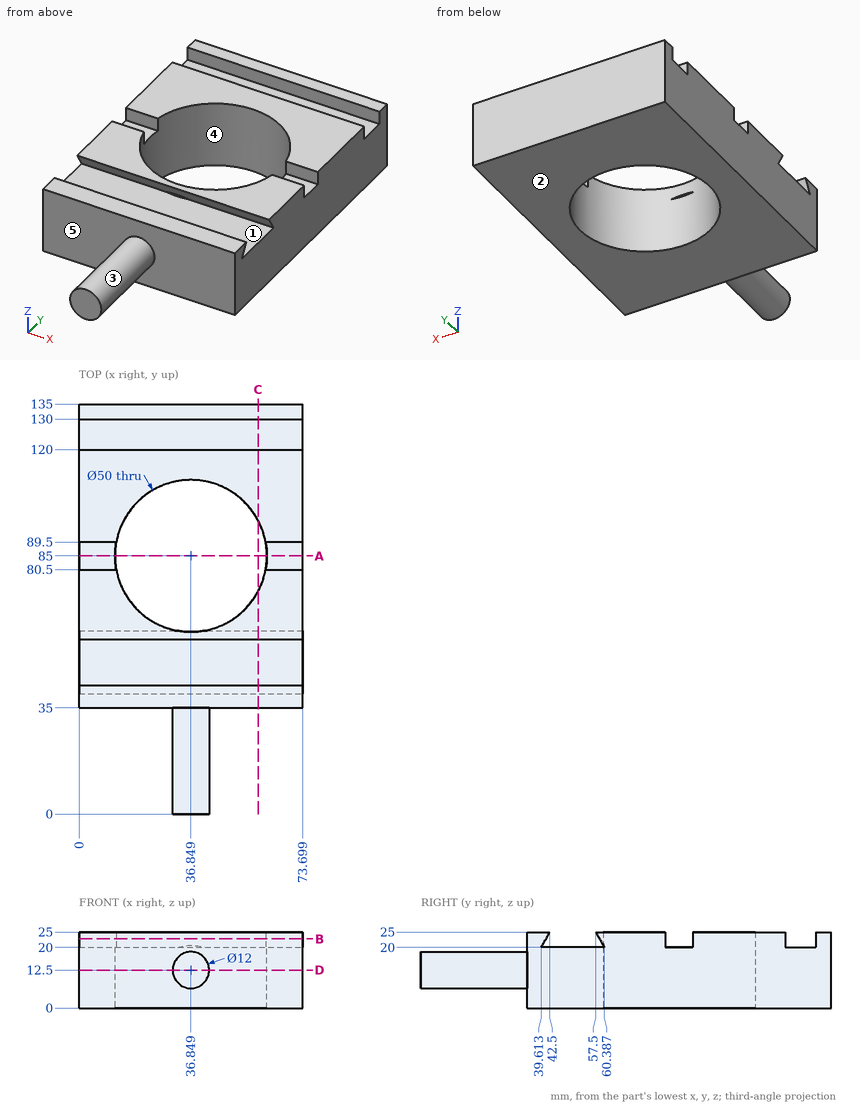
Drawing for the job (mm, zero at the part's lowest x, y, z). A direction names the side the tool comes from. Round coordinates to 2 decimals unless told otherwise and drop trailing zeros. Loops run counter-clockwise (first coordinate to the right, second up) from the corner with the lowest first, then second, coordinate; pieces in that order, holes last. Notation, with made-up numbers: M -28,78 L -12,78 A20 cw -12,103 Z; hole C 4,85 d4. An arc over 180 degrees is marked long. Use a Markdown table: item, result. Add a question column.
(1) Pull direction X, two halves, no side cores. Call the marked faces 3, 4 and 5: +X half, -X half, draft (parallel to the pull), parting line (faces both ways), or undercut.
(2) Cut at D-D (z = 12.5). Give the cut face in (x, y), and give its area (3 significant figures).
(3) Flat gauge pins, fed straight in: pin 1 (2.5 mm diameter, centred on x = 69.5, y = 86, fed in from +Z); pin 2 (1.5 mm diameter, centred on x = 5.5, z = 21.5, fed in from -Y). Where does each tip first touch, or does it go through?
(4) Cut at A-A (y = 85). Give the cut face in (x, z).
(5) Which spindle directions (+Z, -Z, +X, -X, +Y, -Y) get a long thin tool onto all of the face, cutting with end or side? Do the marked faces 1 and 2. Say none if no direction does.
(6) Drill centre lines: line 1 (Y direction, x = 18, z = 20.25) (1 decimal); line 2 (Y direction, x = 17.5, z = 20.75) (1 decimal); line 3 (X direction, y = 85, z = 18.25). Where is each one in solid material? Low to high.
(7) Cut at B-B (z = 22.75). Give the cut face in (x, y).
(8) Cut at C-C (x = 59). Give the cut face in (y, z).
Geometry says:
| question | item | result |
|---|---|---|
| 1 | face 3 | parting line |
| 1 | face 4 | undercut |
| 1 | face 5 | draft |
| 2 | outline | M 0,35 L 30.85,35 L 30.85,0 L 42.85,0 L 42.85,35 L 73.7,35 L 73.7,135 L 0,135 Z; hole C 36.85,85 d50 |
| 2 | area | 5,830 mm² |
| 3 | pin 1 | stops at z = 20 |
| 3 | pin 2 | stops at y = 35 |
| 4 | outline | M 0,0 L 11.85,0 L 11.85,20 L 0,20 Z; M 61.85,0 L 73.7,0 L 73.7,20 L 61.85,20 Z |
| 5 | face 1 | +X, -X |
| 5 | face 2 | -Z, +X, -X, +Y, -Y |
| 6 | line 1 | y = 35 to 39.8, 60.2 to 68.6, 101.4 to 120, 130 to 135 |
| 6 | line 2 | y = 35 to 40, 60 to 69.2, 100.8 to 120, 130 to 135 |
| 6 | line 3 | x = 0 to 11.85, 61.85 to 73.7 |
| 7 | outline | M 0,35 L 73.7,35 L 73.7,41.2 L 0,41.2 Z; M 0,58.8 L 73.7,58.8 L 73.7,80.5 L 61.44,80.5 A25 cw 12.26,80.5 L 0,80.5 Z; M 0,89.5 L 12.26,89.5 A25 cw 61.44,89.5 L 73.7,89.5 L 73.7,120 L 0,120 Z; M 0,130 L 73.7,130 L 73.7,135 L 0,135 Z |
| 8 | outline | M 35,0 L 73.41,0 L 73.41,25 L 57.5,25 L 60.39,20 L 39.61,20 L 42.5,25 L 35,25 Z; M 96.59,0 L 135,0 L 135,25 L 130,25 L 130,20 L 120,20 L 120,25 L 96.59,25 Z |
